Design review of the part built by this model. Coordinates are the model's own, in mm. A direction names the side the tool comes from. Give positions to 0.01 mm unless a question says otherwise; leave off trailing zeros. Write each loop counter-clockwise with the first axis right and the second up, starting at its lowest first coordinate (ties: lowest second). Pieces come first, ordered by that corner, then holes. Notation, with made-up numbers: (80, 16.25) - (139, 16.25) arc R25 cw to (139, 44.25) - close; hole circle Ø3 at (11.5, 12.25). An arc over 180 degrees is marked (long way). Use a Markdown table: item, result. Add a question column.
```python
from build123d import *

# Parameters (mm, degrees)
SKETCH1_W           = 150
SKETCH1_H           = 20
BOSS_EXTRUDE1_DEPTH = 10
SKETCH2_R           = 3
CUT_EXTRUDE1_DEPTH  = 10
SKETCH3_W           = 23
SKETCH3_H           = 25
BOSS_EXTRUDE2_DEPTH = 10
SKETCH4_R           = 2.5
CUT_EXTRUDE2_DEPTH  = 480.576193501
BOSS_EXTRUDE4_START = -20
SKETCH5_W           = 10
SKETCH5_H           = 35
BOSS_EXTRUDE4_DEPTH = 53


with BuildPart() as part:
    # Sketch1 → Boss-Extrude1 (new body)
    with BuildSketch(Plane(origin=(0, 0, 0), x_dir=(1, 0, 0), z_dir=(0, 1, 0))):
        with Locations((-2472.770700637, 441.167728238)):
            Rectangle(SKETCH1_W, SKETCH1_H)
    extrude(amount=BOSS_EXTRUDE1_DEPTH)

    # Sketch2 → Cut-Extrude1 (cut)
    with BuildSketch(Plane(origin=(0, 10, 0), x_dir=(1, 0, 0), z_dir=(0, 1, 0))):
        with Locations(Location((-2407.770700637, 441.167728238, 0), (0, 0, 270))):
            Circle(SKETCH2_R)
    extrude(amount=-CUT_EXTRUDE1_DEPTH, mode=Mode.SUBTRACT)

    # Sketch3 → Boss-Extrude2 (add)
    with BuildSketch(Plane.ZY.offset(2547.770700637)):
        with Locations((-442.667728238, 22.5)):
            Rectangle(SKETCH3_W, SKETCH3_H)
    extrude(amount=-BOSS_EXTRUDE2_DEPTH)

    # Sketch4 → Cut-Extrude2 (cut, through all)
    with BuildSketch(Plane.ZY.offset(2547.770700637)):
        with Locations((-448.417728238, 25)):
            Circle(SKETCH4_R)
        with Locations((-438.417728238, 25)):
            Circle(SKETCH4_R)
    extrude(amount=-CUT_EXTRUDE2_DEPTH, mode=Mode.SUBTRACT)

    # Sketch5 → Boss-Extrude4 (add)
    with BuildSketch(Plane.XY.offset(-431.167728238).offset(BOSS_EXTRUDE4_START)):
        with Locations((-2542.770700637, 17.5)):
            Rectangle(SKETCH5_W, SKETCH5_H)
    extrude(amount=-BOSS_EXTRUDE4_DEPTH)


solid = part.part
```
(1) Mouldability with a two-part tool opening along Z and no side actions: class faces 3 (the face through (-2547.771, 17, -467)), 4 (the face through (-2469, 5, -451.168)), 5 (the face through (-2410.7, 5.07, -441.82)) as +Z half, -Z half, draft (parallel to the pull), parting line (faces both ways), or undercut.
(2) Add section C-C (z = -491.5). State the section outline as (x, y) points.
(3) Tool access review of faces 1 (the face through (-2469, 10, -441)), 2 (the face through (-2490, 9, -431.168)): name each direction out of +Z, -Z, +X, -X, +Y, -Y from which nothing blocks a thin tool from reaching the whole face with its end or side.
(4) Add section D-D (y = 31). State the section outline as (x, z) points, and give its area (3 significant figures).
(5) Add section A-A (y = 25). State the section outline as (x, z) points, and give its area (3 significant figures).
(6) Insertion check: pin 1 (7 mm diameter, centred on x = -2407.77, z = -441.17, fed in from +Y); pin 2 (4.5 mm diameter, centred on y = 25, z = -438.42, fed in from +X); pin 3 (10.5 mm diameter, centred on y = 14.5, z = -480, fed in from +X); pin 4 (8 mm diameter, centred on x = -2439.5, y = 5.5, fed in from -Z). Each pin has a flat end and moves straight along its axis. Give the tip position at first contact, or say it passes through.
(7) For line 1 along X through (y, z) = (33, -460.5); line 2 along Y through (x, z) = (-2509, -441.5); line 3 along Z through (x, y) = (-2451.5, 9.5), list the stretches that pass through material, from the lowest coordinate up.
(8) Add section B-B (y = 4). State the section outline as (x, z) points.
Answers follow:
| question | item | result |
|---|---|---|
| 1 | face 3 | draft |
| 1 | face 4 | -Z half |
| 1 | face 5 | undercut |
| 2 | outline | (-2547.77, 0) - (-2537.77, 0) - (-2537.77, 35) - (-2547.77, 35) - close |
| 3 | face 1 | +Z, -Z, +X, +Y |
| 3 | face 2 | +Z, +X, -X, +Y, -Y |
| 4 | outline | (-2547.77, -504.17) - (-2537.77, -504.17) - (-2537.77, -431.17) - (-2547.77, -431.17) - close |
| 4 | area | 730 mm^2 |
| 5 | outline | (-2547.77, -504.17) - (-2537.77, -504.17) - (-2537.77, -450.92) - (-2547.77, -450.92) - close; (-2547.77, -445.92) - (-2537.77, -445.92) - (-2537.77, -440.92) - (-2547.77, -440.92) - close; (-2547.77, -435.92) - (-2537.77, -435.92) - (-2537.77, -431.17) - (-2547.77, -431.17) - close |
| 5 | area | 630 mm^2 |
| 6 | pin 1 | y = 10 |
| 6 | pin 2 | through |
| 6 | pin 3 | x = -2537.77 |
| 6 | pin 4 | z = -451.17 |
| 7 | line 1 | -2547.77 to -2537.77 |
| 7 | line 2 | 0 to 10 |
| 7 | line 3 | -451.17 to -431.17 |
| 8 | outline | (-2547.77, -504.17) - (-2537.77, -504.17) - (-2537.77, -451.17) - (-2397.77, -451.17) - (-2397.77, -431.17) - (-2547.77, -431.17) - close; hole circle Ø6 at (-2407.77, -441.17) |
